Input: part model. Units: mm. Frame: model coordinates. A direction names the side the tool comes from. Round coordinates to 2 decimals unless told otherwise and drop trailing zeros. Loops run counter-clockwise (first coordinate to the right, second up) from the corner with the lowest first, then second, coordinate; pieces in that order, holes last.
1) First-contact query: pin 1 (3.5 mm diameter, centred on x = 0, y = 0, fed in from +Z); pin 2 (10 mm diameter, centred on y = -70.5, z = -9, fed in from -X); pin 3 (8 mm diameter, centred on x = 11, y = -82.5, fed in from +Z). Flat tips, straight axial feed; report the tip coordinate or a pass-through.
2) Section C-C, the plane x = 33.5. Return loops of the section in (y, z).
3) Section A-A, the plane z = -5.5. Return loops of the section in (x, y), and give its area (3 significant figures).
4) Section B-B, the plane y = 0. Return loops of the section in (x, z), and give its area (3 significant figures).
5) Ray query, line 1 along Y through (x, z) = (51.5, 9); line 2 along Y through (x, z) = (0, -6.1); line 3 along Y through (x, z) = (-19, 10). Return the intervals inside material, ascending.
6) Section D-D, the plane z = 2.5. Return loops of the section in (x, y).
7) Access query for faces 4 (the face through (0, -55, -10)), 5 (the face through (-57.94, -18.48, 15.56)), 6 (the face through (-3, 0, -5)). Directions: +Z, -Z, +X, -X, +Y, -Y. A direction counts if a zero-diameter tool reaches every point of the face in a straight line with its end or side. Return the directions, or none.
8) Draft query along Y for faces 1 (the face through (0, 13, 12)), 2 (the face through (-1, -19.05, 3)), 3 (the face through (1.3, -1.3, -7)). Return one class per face: pulls with the +Y half, pulls with the -Y half, needs draft (parallel to the pull), parting line crosses it, or undercut.
from build123d import *

# Parameters (mm, degrees)
F1_DEPTH  = 19.05
F2_R      = 63.5
F3_DEPTH  = 6.35
F4_R      = 2
F5_R      = 1.5
F6_DEPTH  = 33.001
F7_R      = 3
F8_DEPTH  = 7
F9_W      = 20
F9_H      = 3
F10_DEPTH = 75
F12_DEPTH = 3.001
F13_F1_R  = 2
F13_F2_R  = 2


with BuildPart() as f1:
    # F0 (on Front) → F1 (new body, symmetric)
    with BuildSketch(Plane.XZ):
        with BuildLine():
            Line((-70, -13), (70, -13))
            Line((70, -13), (70, 12))
            Line((70, 12), (47, 20))
            Line((47, 20), (26.6833281283, 20))
            ThreePointArc((26.6833281283, 20), (0, 12), (-26.6833281283, 20))
            Line((-26.6833281283, 20), (-47, 20))
            Line((-47, 20), (-70, 12))
            Line((-70, 12), (-70, -13))
        make_face()
    extrude(amount=F1_DEPTH, both=True)

    # F2 (on Front) → F3 (cut, symmetric)
    with BuildSketch(Plane.XZ):
        with Locations((0, 60.5)):
            Circle(F2_R)
    extrude(amount=F3_DEPTH, both=True, mode=Mode.SUBTRACT)

    # F4
    f4_edges = [f1.edges().sort_by_distance(p)[0] for p in [
        (-70, -19.05, -0.5),
        (-58.5, -19.05, 16),
        (-36.841664, -19.05, 20),
        (0, -19.05, 12),
        (36.841664, -19.05, 20),
        (58.5, -19.05, 16),
        (70, -19.05, -0.5),
        (70, 0, 12),
        (47, -12.7, 20),
        (26.683328, -12.7, 20),
        (26.683328, 12.7, 20),
        (47.738913, -6.35, 19.742987),
        (48.477826, 0, 19.485974),
        (47.738913, 6.35, 19.742987),
        (47, 12.7, 20),
        (58.5, 19.05, 16),
        (70, 19.05, -0.5),
        (0, 6.35, 12),
        (-26.683328, 12.7, 20),
        (0, 19.05, 12),
        (-26.683328, -12.7, 20),
        (0, -6.35, 12),
        (-47, -12.7, 20),
        (-36.841664, -6.35, 20),
        (-36.841664, 6.35, 20),
        (-47, 12.7, 20),
        (-36.841664, 19.05, 20),
        (-47.738913, 6.35, 19.742987),
        (-48.477826, 0, 19.485974),
        (-47.738913, -6.35, 19.742987),
        (-70, 0, 12),
        (-58.5, 19.05, 16),
        (-70, 19.05, -0.5),
        (36.841664, 6.35, 20),
        (36.841664, 19.05, 20),
        (36.841664, -6.35, 20),
    ]]
    fillet(f4_edges, radius=F4_R)

    # F5 (on face) → F6 (cut, through all)
    with BuildSketch(Plane(origin=(0, 0, -13), x_dir=(1, 0, 0), z_dir=(0, 0, -1))):
        Circle(F5_R)
    extrude(amount=-F6_DEPTH, mode=Mode.SUBTRACT)

    # F7 (on Top) → F8 (cut)
    with BuildSketch(Plane.XY):
        Circle(F7_R)
    extrude(amount=-F8_DEPTH, mode=Mode.SUBTRACT)

    # F9 (on face) → F10 (join)
    with BuildSketch(Plane.XZ.offset(19.05)):
        with Locations((0, -11.5)):
            Rectangle(F9_W, F9_H)
    extrude(amount=F10_DEPTH)

    # F11 (on face) → F12 (cut, through all)
    with BuildSketch(Plane.XY.offset(-10)):
        Polygon((-10, -94.05), (0, -94.05), (-10, -79.05), align=None)
        Polygon((10, -79.05), (0, -94.05), (10, -94.05), align=None)
    extrude(amount=-F12_DEPTH, mode=Mode.SUBTRACT)

    # F13: fillet of radius 2 on 5 edges, made by hand

    # F13_f1
    f13_f1_edges = [f1.edges().sort_by_distance(p)[0] for p in [
        (-10, -49.05, -10),
        (-5, -86.55, -10),
        (5, -86.55, -10),
        (10, -49.05, -10),
    ]]
    fillet(f13_f1_edges, radius=F13_F1_R)

    # F13_f2
    f13_f2_edges = [f1.edges().sort_by_distance(p)[0] for p in [
        (0, -19.05, -10),
        (9.4142135624, -19.05, -10.5857864376),
        (-9.4142135624, -19.05, -10.5857864376),
    ]]
    fillet(f13_f2_edges, radius=F13_F2_R)


solid = f1.part
Final values:
1. pin 1: stops at z = -7
1. pin 2: stops at x = -10
1. pin 3: stops at z = -10.14
2. outline: (-19.05, -13) - (19.05, -13) - (19.05, 18) arc R2 ccw to (17.05, 20) - (8.35, 20) arc R2 ccw to (6.35, 18) - (6.35, 6.56) - (-6.35, 6.56) - (-6.35, 18) arc R2 ccw to (-8.35, 20) - (-17.05, 20) arc R2 ccw to (-19.05, 18) - close
3. outline: (-70, -17.05) arc R2 ccw to (-68, -19.05) - (68, -19.05) arc R2 ccw to (70, -17.05) - (70, 17.05) arc R2 ccw to (68, 19.05) - (-68, 19.05) arc R2 ccw to (-70, 17.05) - close; hole circle Ø6 at (0, 0)
3. area: 5,300 mm2
4. outline: (-70, -13) - (-1.5, -13) - (-1.5, -7) - (-3, -7) - (-3, -2.93) arc R63.5 cw to (-47.6, 18.47) arc R2 ccw to (-49.76, 19.04) - (-68.66, 12.47) arc R2 ccw to (-70, 10.58) - close; (1.5, -13) - (70, -13) - (70, 10.58) arc R2 ccw to (68.66, 12.47) - (49.76, 19.04) arc R2 ccw to (47.6, 18.47) arc R63.5 cw to (3, -2.93) - (3, -7) - (1.5, -7) - close
4. area: 2,830 mm2
5. line 1: y = -19.05 to 19.05
5. line 2: y = -19.05 to -3, 3 to 19.05
5. line 3: y = -19.05 to -6.35, 6.35 to 19.05
6. outline: (-70, -17.05) arc R2 ccw to (-68, -19.05) - (68, -19.05) arc R2 ccw to (70, -17.05) - (70, 17.05) arc R2 ccw to (68, 19.05) - (-68, 19.05) arc R2 ccw to (-70, 17.05) - close; hole (-25.85, -6.35) - (25.85, -6.35) - (25.85, 6.35) - (-25.85, 6.35) - close
7. face 4: +Z, +X, -X, -Y
7. face 5: +Z, -X, -Y
7. face 6: +Z
8. face 1: needs draft
8. face 2: pulls with the -Y half
8. face 3: undercut
